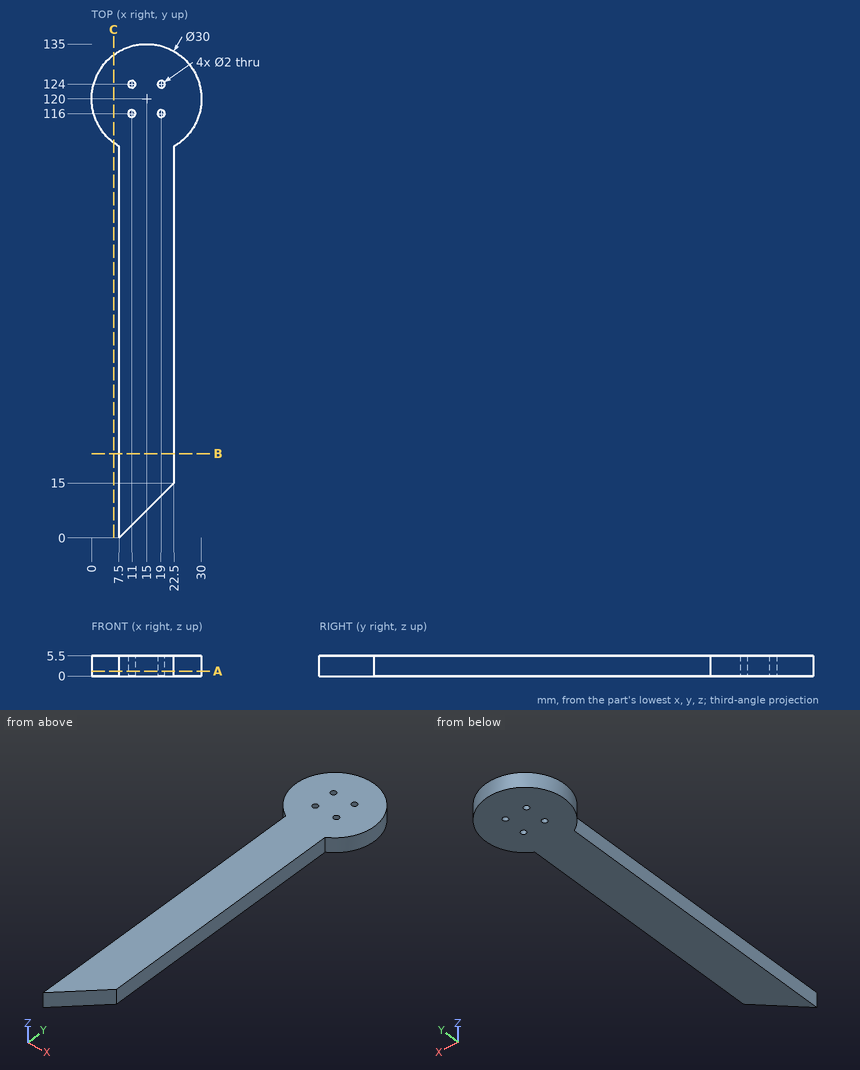
Can you work these out from the drawing? Everything is in mm from the part's minimum corner. Give positions to 0.01 mm unless a question says otherwise; leave off trailing zeros. Loops run counter-clockwise (first coordinate to the right, second up) from the corner with the lowest first, then second, coordinate; pieces in that order, holes last. Notation, with made-up numbers: (-39.5, 2.25) - (-35.5, 2.25) arc R18 cw to (-35.5, 11.25) - close; hole circle Ø3 at (49.5, 76.5). An arc over 180 degrees is marked (long way). Answer as a JSON object with one key per item and string values.
Q1. Imagine slicing it at B-B on y = 23. Write out the boundary of the cut face in (x, z), plus the area to 3 significant figures.
Geometry says:
{"outline": "(7.5, 0) - (22.5, 0) - (22.5, 5.5) - (7.5, 5.5) - close", "area": "82.5 mm²"}
Q2. If I drill on L1, parallel to X at y = 116, z = 1.4; L2, parallel to Y at x = 11, z = 3.1; L3, parallel to X at y = 44.5, z = 4.9, over which ranges is the centre line in solid material (lowest first)?
Geometry says:
{"L1": "0.54 to 10, 12 to 18, 20 to 29.46", "L2": "3.5 to 115, 117 to 123, 125 to 134.46", "L3": "7.5 to 22.5"}
Q3. Will these pins go through, and if not, where does the flat tip stop? P1, Ø1.6, axis at y = 42, z = 2.5, coming from the +X side; P2, Ø3, axis at y = 58.5, z = 2, coming from the -X side; P3, Ø1, axis at x = 4.5, z = 3.5, coming from the +Y side; P4, Ø1.8, axis at x = 11, y = 116, coming from the -Z side.
Geometry says:
{"P1": "x = 22.5", "P2": "x = 7.5", "P3": "y = 131.18", "P4": "through"}
Q4. Imagine slicing it at A-A on z = 1.3. Write out the boundary of the cut face in (x, y), plus the area to 3 significant figures.
Geometry says:
{"outline": "(7.5, 0) - (22.5, 15) - (22.5, 107.01) arc R15 ccw (long way) to (7.5, 107.01) - close; hole circle Ø2 at (11, 116); hole circle Ø2 at (11, 124); hole circle Ø2 at (19, 116); hole circle Ø2 at (19, 124)", "area": "2,170 mm²"}
Q5. Imagine slicing it at C-C on x = 6. Write out the boundary of the cut face in (y, z), plus the area to 3 significant figures.
Geometry says:
{"outline": "(108, 0) - (132, 0) - (132, 5.5) - (108, 5.5) - close", "area": "132 mm²"}
